Input: part model. Units: mm. Frame: model coordinates. Round coordinates to 2 decimals unless told otherwise and drop trailing zeros. Write each loop counter-clockwise with the first axis right and the second up, starting at its lowest first coordinate (ties: lowest second). Pieces come first, ordered by that corner, then holes. Notation, with made-up numbers: (50, -35.75) -> (58, -35.75) arc R9 cw to (58, -22.75) -> close; hole circle Ø3 at (7.25, 2.5). An arc over 180 degrees is marked (long way). Write item = value, one per line. Start each with the question number.
```python
from build123d import *

# Parameters (mm, degrees)
SKETCH1_R      = 19.05
EXTRUDE1_DEPTH = 38.1
CHAMFER1_SIZE  = 0.762


with BuildPart() as part:
    # Sketch1 → Extrude1 (new body)
    with BuildSketch(Plane(origin=(0, 0, 0), x_dir=(1, 0, 0), z_dir=(0, 1, 0))):
        with Locations(Location((0, 0, 0), (0, 0, 270))):  # turned: the seam where the file's is
            Circle(SKETCH1_R)
    extrude(amount=EXTRUDE1_DEPTH)

    # Sketch2 → 3/4 (0.75) Diameter Hole1 (revolve, cut)
    with BuildSketch(Plane(origin=(0, 38.1, 0), x_dir=(0, 0, 1), z_dir=(1, 0, 0))):
        Polygon((0, 0), (0, 38.1), (10.16, 38.1), (9.525, 37.465), (9.525, 0.635), (10.16, 0), align=None)
    revolve(axis=Axis((0, 44.45, 0), (0, -1, 0)), mode=Mode.SUBTRACT)

    # Chamfer1
    chamfer1_edges = [part.edges().sort_by_distance(p)[0] for p in [
        (0, 0, -19.05),
        (0, 38.1, -19.05),
    ]]
    chamfer(chamfer1_edges, length=CHAMFER1_SIZE)


solid = part.part
```
1. Section C-C (y = 10). Output: boundary loops of the cut face in (x, z) (3 decimals), then the cut area to 3 significant figures.
2. Section B-B (z = 0). Output: boundary loops of the cut face in (x, y) (3 decimals), then the cut area to 3 significant figures.
3. Pin query (flat end, axial travel): P1, Ø3, axis at x = -11, y = 10.5, coming from the +Z side; P2, Ø3, axis at y = 23, z = 3.5, coming from the -X side; P3, Ø3, axis at y = 17, z = 1.5, coming from the +X side. Return the tip coordinate at first contact, or that it passes through.
4. Mould query, pull axis Z, two halves, no side actions, for faces 1 (the flat face through (-8, 38.1, 8)), 2 (the cylindrical face through (5.796, 19.308, -7.559)), 3 (the cylindrical face through (-11.59, 18.79, -15.12)). Classes: pulls with the +Z half, pulls with the -Z half, needs draft (parallel to the pull), parting line crosses it, or undercut.
5. Line query: line 1 along X through (y, z) = (14, 0) (3 decimals); line 2 along Z through (x, y) = (1, 27); line 3 along X through (y, z) = (34, 2.5). Output: solid intervals per line, ascending.
6. Section A-A (x = 0). Output: boundary loops of the cut face in (y, z) (3 decimals).
Check sheet entries:
q1.outline = circle Ø38.1 at (0, 0); hole circle Ø19.05 at (0, 0)
q1.area = 855 mm2
q2.outline = (-19.05, 0.762) -> (-18.288, 0) -> (-10.16, 0) -> (-9.525, 0.635) -> (-9.525, 37.465) -> (-10.16, 38.1) -> (-18.288, 38.1) -> (-19.05, 37.338) -> close; (9.525, 0.635) -> (10.16, 0) -> (18.288, 0) -> (19.05, 0.762) -> (19.05, 37.338) -> (18.288, 38.1) -> (10.16, 38.1) -> (9.525, 37.465) -> close
q2.area = 724 mm2
q3.P1 = 16.51
q3.P2 = -18.94
q3.P3 = 19.05
q4.face_1 = needs draft
q4.face_2 = undercut
q4.face_3 = parting line crosses it
q5.line_1 = -19.05 to -9.525, 9.525 to 19.05
q5.line_2 = -19.02 to -9.47, 9.47 to 19.02
q5.line_3 = -18.89 to -9.19, 9.19 to 18.89
q6.outline = (0, -18.288) -> (0.762, -19.05) -> (37.338, -19.05) -> (38.1, -18.288) -> (38.1, -10.16) -> (37.465, -9.525) -> (0.635, -9.525) -> (0, -10.16) -> close; (0, 10.16) -> (0.635, 9.525) -> (37.465, 9.525) -> (38.1, 10.16) -> (38.1, 18.288) -> (37.338, 19.05) -> (0.762, 19.05) -> (0, 18.288) -> close
